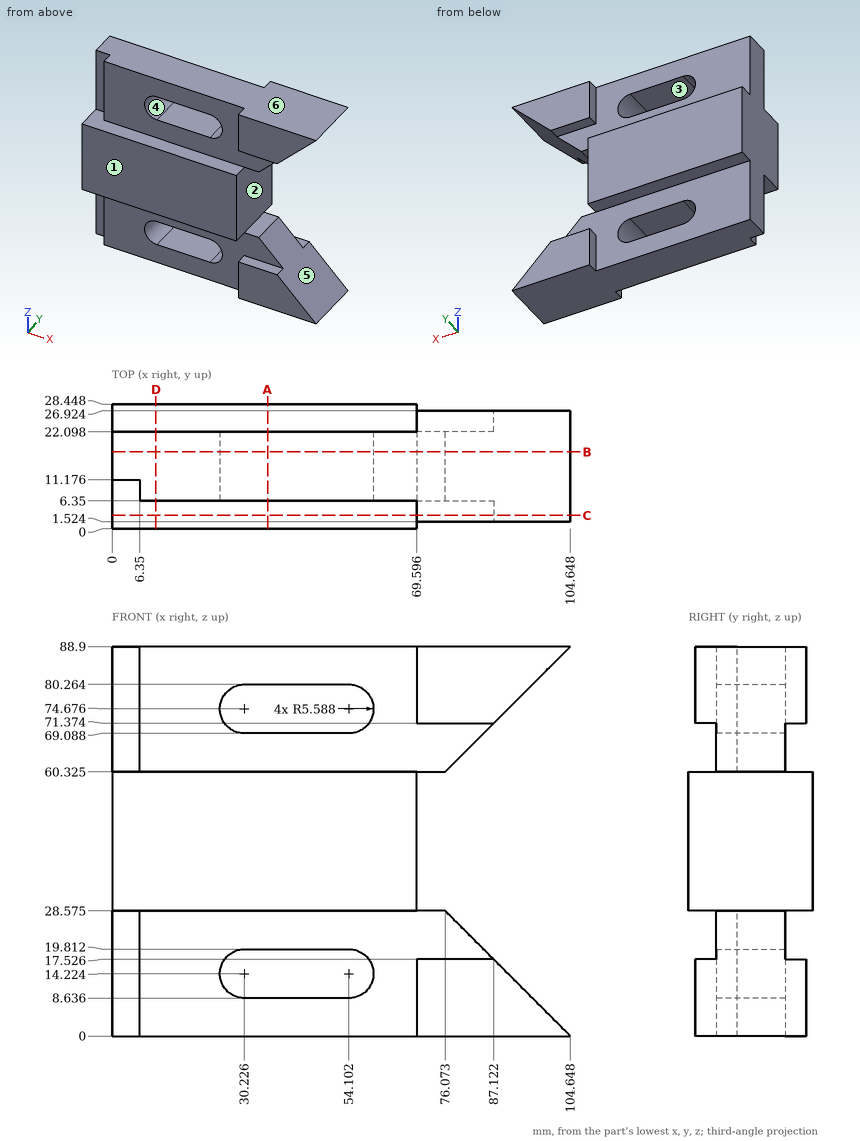
Input: dimensioned drawing with shaded views. Units: mm. Origin: part minimum x, y, z. A direction names the side the tool comes from. Give positions to 0.01 mm unless a question says otherwise; leave off trailing zeros. Write each loop counter-clockwise with the first axis right and the second up, starting at its lowest first coordinate (ties: lowest second). Pieces come first, ordered by that corner, then holes. Notation, with made-up numbers: M 44.25,72.5 L 83.25,72.5 A32 cw 83.25,110.5 Z; hole C 23,-4 d3. An arc over 180 degrees is marked long. Write item = value, one per line. Start each with the question number.
1) Cut plane C-C on y = 3. Return the cut outline in (x, z) (3 decimals), then the cut area to 3 significant figures.
2) Material intervals for line 1 along Z through (x, y) = (44, 14.25); line 2 along Z through (x, y) = (73, 12.5) (3 decimals); line 3 along Y through (x, z) = (14.5, 12), sorted ascending. Write a range as [from, to].
3) First-contact query: pin 1 Ø3 at (x, y) = (32.5, 25.5) entering from -Z (3 decimals); pin 2 Ø5 at (x, z) = (4.5, 21) entering from -Y; pin 3 Ø19.5 at (x, z) = (93, 10.5) entering from -Y. Flat tips, straight axial feed; report the tip coordinate or a pass-through.
4) Reachability of the marked faces 4, 5 and 6 from +Z, -Z, +X, -X, +Y, -Y: full face, straight path, thin tool, end or side. Return the list, or none.
5) Cut plane D-D on x = 10. Return the cut outline in (y, z) (3 decimals), then the cut area to 3 significant figures.
6) Draft query along X for the marked faces 1, 2 and 3. Return one class per face: +X half, -X half, draft (parallel to the pull), parting line (faces both ways), or undercut.
7) Cut plane B-B on y = 17.5. Return the cut outline in (x, z) (3 decimals).
8) Cut plane A-A on x = 35.5. Return the cut outline in (y, z) (3 decimals), then the cut area to 3 significant figures.
Solved:
q1.outline = M 0,28.575 L 69.596,28.575 L 69.596,60.325 L 0,60.325 Z; M 69.596,0 L 104.648,0 L 87.122,17.526 L 69.596,17.526 Z; M 69.596,71.374 L 87.122,71.374 L 104.648,88.9 L 69.596,88.9 Z
q1.area = 3,130 mm2
q2.line_1 = [0, 8.64], [19.81, 69.09], [80.26, 88.9]
q2.line_2 = [0, 28.575], [60.325, 88.9]
q2.line_3 = [6.35, 22.1]
q3.pin_1 = 28.575
q3.pin_2 = 6.35
q3.pin_3 = 1.52
q4.face_4 = +Y, -Y
q4.face_5 = +X, +Y, -Y
q4.face_6 = +Z, +X, -X, +Y, -Y
q5.outline = M 0,28.575 L 6.35,28.575 L 6.35,0 L 22.098,0 L 22.098,28.575 L 28.448,28.575 L 28.448,60.325 L 22.098,60.325 L 22.098,88.9 L 6.35,88.9 L 6.35,60.325 L 0,60.325 Z
q5.area = 1,800 mm2
q6.face_1 = draft
q6.face_2 = +X half
q6.face_3 = undercut
q7.outline = M 0,0 L 104.648,0 L 76.073,28.575 L 69.596,28.575 L 69.596,60.325 L 76.073,60.325 L 104.648,88.9 L 0,88.9 Z; hole M 30.226,8.636 L 54.102,8.636 A5.588 ccw 54.102,19.812 L 30.226,19.812 A5.588 ccw Z; hole M 30.226,69.088 L 54.102,69.088 A5.588 ccw 54.102,80.264 L 30.226,80.264 A5.588 ccw Z
q8.outline = M 0,28.575 L 6.35,28.575 L 6.35,19.812 L 22.098,19.812 L 22.098,28.575 L 28.448,28.575 L 28.448,60.325 L 22.098,60.325 L 22.098,69.088 L 6.35,69.088 L 6.35,60.325 L 0,60.325 Z; M 6.35,0 L 22.098,0 L 22.098,8.636 L 6.35,8.636 Z; M 6.35,80.264 L 22.098,80.264 L 22.098,88.9 L 6.35,88.9 Z
q8.area = 1,450 mm2
